Geometry check sheet. Reference: the model listing, model coordinates, mm. A direction names the side the tool comes from. Round coordinates to 2 decimals unless told otherwise and drop trailing zeros. Loops run counter-clockwise (first coordinate to the right, second up) from the corner with the lowest first, then second, coordinate; pieces in that order, holes last. Notation, with made-up numbers: (51.5, 71.5) -> (74.5, 71.5) arc R21 cw to (74.5, 88.5) -> close; hole circle Ø9 at (-25, -14). An arc over 180 degrees is marked (long way). Use one line per item in the form item = value.
from build123d import *

# Parameters (mm, degrees)
SKETCH1_R           = 1.5
BOSS_EXTRUDE1_DEPTH = 1.5
SKETCH2_R           = 4.5
BOSS_EXTRUDE2_DEPTH = 100
FILLET2_R           = 1.5


with BuildPart() as part:
    # Sketch1 → Boss-Extrude1 (new body)
    with BuildSketch(Plane(origin=(0, 0, 0), x_dir=(1, 0, 0), z_dir=(0, 1, 0))):
        with BuildLine():
            Line((5.75, 9), (-5.75, 9))
            ThreePointArc((-5.75, 9), (-8.048097039, 8.048097039), (-9, 5.75))
            Line((-9, 5.75), (-9, -5.75))
            ThreePointArc((-9, -5.75), (-8.048097039, -8.048097039), (-5.75, -9))
            Line((-5.75, -9), (5.75, -9))
            ThreePointArc((5.75, -9), (8.048097039, -8.048097039), (9, -5.75))
            Line((9, -5.75), (9, 5.75))
            ThreePointArc((9, 5.75), (8.048097039, 8.048097039), (5.75, 9))
        make_face()
        with Locations((5.75, 5.75)):
            Circle(SKETCH1_R, mode=Mode.SUBTRACT)
        with Locations((5.75, -5.75)):
            Circle(SKETCH1_R, mode=Mode.SUBTRACT)
        with Locations((-5.75, -5.75)):
            Circle(SKETCH1_R, mode=Mode.SUBTRACT)
        with Locations((-5.75, 5.75)):
            Circle(SKETCH1_R, mode=Mode.SUBTRACT)
    extrude(amount=BOSS_EXTRUDE1_DEPTH)

    # Sketch2 → Boss-Extrude2 (add)
    with BuildSketch(Plane(origin=(0, 1.5, 0), x_dir=(1, 0, 0), z_dir=(0, 1, 0))):
        Circle(SKETCH2_R)
    extrude(amount=BOSS_EXTRUDE2_DEPTH)

    # Fillet2
    fillet2_edges = [part.edges().sort_by_distance(p)[0] for p in [
        (-4.5, 1.5, 0),
    ]]
    fillet(fillet2_edges, radius=FILLET2_R)


solid = part.part
1. Material ranges on line 1 along Z through (x, y) = (-5.75, 0.8); line 2 along Y through (x, z) = (-0.5, 6), recorded low to high.
Return value:
line_1 = -9 to -7.25, -4.25 to 4.25, 7.25 to 9
line_2 = 0 to 1.5
2. Section check B-B (z = 0). Record the boundary of the cut face in (x, y), then the cut area to 3 significant figures.
Return value:
outline = (-9, 0) -> (9, 0) -> (9, 1.5) -> (6, 1.5) arc R1.5 cw to (4.5, 3) -> (4.5, 101.5) -> (-4.5, 101.5) -> (-4.5, 3) arc R1.5 cw to (-6, 1.5) -> (-9, 1.5) -> close
area = 928 mm2
3. Gauge pin test, flat ends, axial feed: pin 1 (8 mm diameter, centred on y = 86, z = 6, fed in from -X); pin 2 (8 mm diameter, centred on x = 6.5, y = 59.5, fed in from -Z); pin 3 (4 mm diameter, centred on y = 53.5, z = -1.5, fed in from +X). Record the tip position at first contact, or that the pin passes through.
Return value:
pin_1 = -4.03
pin_2 = -3.74
pin_3 = 4.5
4. Section check C-C (y = 23.5). Record the boundary of the cut face in (x, z), then the cut area to 3 significant figures.
Return value:
outline = circle Ø9 at (0, 0)
area = 63.6 mm2
5. Section check A-A (x = 0). Record the boundary of the cut face in (y, z), then the cut area to 3 significant figures.
Return value:
outline = (0, -9) -> (1.5, -9) -> (1.5, -6) arc R1.5 cw to (3, -4.5) -> (101.5, -4.5) -> (101.5, 4.5) -> (3, 4.5) arc R1.5 cw to (1.5, 6) -> (1.5, 9) -> (0, 9) -> close
area = 928 mm2
6. Tool access check on faces 4 (the flat face through (2, 1.5, 6)), 5 (the flat face through (0, 0, 0)). Record the directions out of +Z, -Z, +X, -X, +Y, -Y that give a thin tool (end or side, any length) a straight path to the whole face; none if there is none.
Return value:
face_4 = +Y
face_5 = +Z, -Z, +X, -X, -Y
7. Mould release check, pull along X, two halves, no side actions. Record for faces 1 (the flat face through (0, 101.5, 0)), 2 (the cylindrical face through (4.56, 0.74, -4.84)), 3 (the cylindrical face through (-0.59, 51.56, -4.46)): released by +X, released by -X, zero draft, split by the parting line, or undercut.
Return value:
face_1 = zero draft
face_2 = undercut
face_3 = split by the parting line
